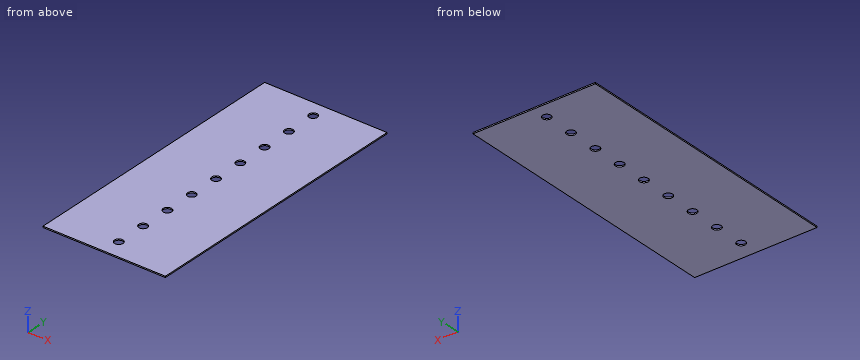
Autodesk Inventor part; units mm, degrees
ref_plane "YZ Plane" through (0, 0, 0) normal (1, 0, 0) x (0, 1, 0)
ref_plane "XZ Plane" through (0, 0, 0) normal (0, 1, 0) x (-1, 0, 0)
ref_plane "XY Plane" through (0, 0, 0) normal (0, 0, 1) x (1, 0, 0)
sketch "Sketch1" plane through (0, 0, 0) normal (0, 0, 1) x (1, 0, 0)
  line L0 (-500, -1140) -> (500, -1140)
  line L1 (500, -1140) -> (500, 1140)
  line L2 (500, 1140) -> (-500, 1140)
  line L3 (-500, 1140) -> (-500, -1140)
  line L4 (-500, -1140) -> (500, 1140) construction
  line L5 (500, -1140) -> (-500, 1140) construction
  point P0 (0, 0)
  dimension "d0" = 1000
  dimension "d1" = 2280
extrude "Plate1" add sketch "Sketch1" along normal blind 10
sketch "Sketch2" plane through (0, 0, 10) normal (0, 0, 1) x (1, 0, 0)
  line L0 (500, -1140) -> (-500, -1140)
  line L1 (500, 1140) -> (500, -1140)
  line L2 (-500, 1140) -> (500, 1140)
  line L3 (-500, -1140) -> (-500, 1140)
  circle A0 centre (0, -989.5) radius 35
  point P0 (0, 0)
  point P1 (0, -1140)
  dimension "d3" = 70
  dimension "d4" = 150.5
extrude "Extrusion1" cut sketch "Sketch2" against normal through all contours A0
pattern_linear "Rectangular Pattern1" count 9 spacing 250 along (0, 1, 0) of "Extrusion1"
equation "\"d2\" = Thickness"
equation "\"BendReliefDepth\" = 0.5 * Thickness"
properties part number "ДМФ 067 крышка"
Source: CAD feature listing. Evaluate the final solid. Frame: model axes, mm. Coordinates: 2 decimals unless noted, no trailing zeros. Loops run counter-clockwise (first coordinate to the right, second up) from the corner with the lowest first, then second, coordinate; pieces in that order, holes last. Notation, with made-up numbers: (27.25, -26.5) -> (35.25, -26.5) arc R7 cw to (35.25, -13.5) -> close; hole circle Ø5 at (26.5, -15). An arc over 180 degrees is marked (long way). One line per item, written item: value. Start each with the question number.
Q1. Line query: line 1 along X through (y, z) = (-505.5, 6.5). Output: solid intervals per line, ascending.
Q2. Section query A-A, the plane y = -989.5. Return the cut outline in (x, z), and give its area (3 significant figures).
Q3. Contact query for a flat-ended pin moving along its axis: P1, Ø6, axis at x = -68, y = 823.5, coming from the -Z side. Output: stop coordinate, or through.
Q4. Section query B-B, the plane z = 3.25. Give the number of separate pieces and of enclosed holes in the cut face, and give its area (3 significant figures).
Results:
1. line 1: -500 to -31.13, 31.13 to 500
2. outline: (-500, 0) -> (-35, 0) -> (-35, 10) -> (-500, 10) -> close; (35, 0) -> (500, 0) -> (500, 10) -> (35, 10) -> close
2. area: 9,300 mm^2
3. P1: z = 0
4. separate pieces: 1
4. enclosed holes: 9
4. area: 2,250,000 mm^2
